The model under review builds one solid part; all positions refer to its coordinate system, in mm. A direction names the side the tool comes from. Give positions to 0.01 mm unless a question says otherwise; leave off trailing zeros. Order: outer loops, then holes, each group sorted by start corner. A loop starts at its lowest first (then second) coordinate and runs counter-clockwise, first axis right, second up. Notation, with made-up numbers: (54, 10) - (70, 10) arc R23 cw to (70, 32) - close; hole circle Ø4 at (-35.75, -19). An arc over 180 degrees is marked (long way). Write item = value, one per line. Start each with the question number.
1. Mouldability with a two-part tool opening along X and no side actions: class faces 4 (the flat face through (0, 0, 0)), 5 (the cylindrical face through (3.612, -3.312, 22.185)), 6 (the conical face through (-2.545, -1.372, 8.397)) as pulls with the +X half, pulls with the -X half, needs draft (parallel to the pull), parting line crosses it, or undercut.
2. We need section A-A, the plane z = 35. Give the boundary of the cut face in (x, y).
3. We need section D-D, the plane z = 5. Give the boundary of the cut face in (x, y).
4. We need section B-B, the plane z = 19. Give the boundary of the cut face in (x, y).
5. For P1, Ø2, axis at x = 2.5, y = 3.5, coming from the -Z side; P2, Ø1.4, axis at x = -2.6, y = -1.5, coming from the -Z side; P3, Ø1, axis at y = -4, z = 29, coming from the +X side; P4, Ø3.5, axis at x = 0, y = 0, coming from the +Z side, all flat-tipped, find the tip position at first contact; note any pin that passes through.
6. Machinability: for faces 1 (the cylindrical face through (-0.631, -2.003, 38.098)), 2 (the flat face through (-2.1, 1, 45)), 3 (the cylindrical face through (3.308, -1.131, 3.944)), which of the approach directions +Z, -Z, +X, -X, +Y, -Y give a long, thin tool a straight path to every point of the face, cutting with its end or side? Answer none if there is none.
7. Wall thickness on probe 1 along Y at (x, z) = (0, 4.25); probe 2 along X at (y, z) = (-1.75, 6); probe 3 along X at (y, z) = (3, 4): over which ranges is each line inside the solid? List them lowest first.
8. We need section C-C, the plane y = -3.25. Give the boundary of the cut face in (x, z).
from build123d import *

# Parameters (mm, degrees)
ESBO_O1_R                = 4.9
RESSALTO_EXTRUS_O1_DEPTH = 45
PADR_OCIRCULAR1_COUNT    = 3


with BuildPart() as part:
    # Esboço1 → Ressalto-extrusão1 (new body)
    with BuildSketch(Plane.XY):
        with Locations(Location((0, 0, 0), (0, 0, 180))):
            Circle(ESBO_O1_R)
    extrude(amount=RESSALTO_EXTRUS_O1_DEPTH)

    # Esboço2 → Furo roscado de M51 (revolve, cut)
    with BuildSketch(Plane(origin=(0, 0, 45), x_dir=(0, -1, 0), z_dir=(1, 0, 0))):
        Polygon((0, 0), (0, 15.2618073), (2.1, 14), (2.1, 0), align=None)
    revolve(axis=Axis((0, 0, 51.35), (0, 0, -1)), mode=Mode.SUBTRACT)

    # Esboço6 → Furo roscado de M21 (revolve, cut)
    with BuildSketch(Plane(origin=(0, 3, 0), x_dir=(0, 1, 0), z_dir=(1, 0, 0))):
        Polygon((0, 0), (0, 8.480688495), (0.8, 8), (0.8, 0), align=None)
    furo_roscado_de_m21 = revolve(axis=Axis((0, 3, -6.35), (0, 0, 1)), mode=Mode.SUBTRACT)

    # PadrãoCircular1: Furo roscado de M21 ×3 about axis
    padr_ocircular1_axis = Axis((0, 0, 0), (0, 0, 1))
    for i in range(1, PADR_OCIRCULAR1_COUNT):
        add(furo_roscado_de_m21.rotate(padr_ocircular1_axis, i * 360 / PADR_OCIRCULAR1_COUNT), mode=Mode.SUBTRACT)


solid = part.part
Model answer:
q1.face_4 = needs draft
q1.face_5 = parting line crosses it
q1.face_6 = undercut
q2.outline = circle Ø9.8 at (0, 0); hole circle Ø4.2 at (0, 0)
q3.outline = circle Ø9.8 at (0, 0); hole circle Ø1.6 at (-2.6, -1.5); hole circle Ø1.6 at (0, 3); hole circle Ø1.6 at (2.6, -1.5)
q4.outline = circle Ø9.8 at (0, 0)
q5.P1 = 0
q5.P2 = 8.06
q5.P3 = 3.43
q5.P4 = 30.79
q6.face_1 = +Z
q6.face_2 = +Z, +X, -X, +Y, -Y
q6.face_3 = -Z
q7.probe_1 = -4.9 to 2.2, 3.8 to 4.9
q7.probe_2 = -4.58 to -3.36, -1.84 to 1.84, 3.36 to 4.58
q7.probe_3 = -3.87 to -0.8, 0.8 to 3.87
q8.outline = (-3.67, 0) - (3.67, 0) - (3.67, 45) - (-3.67, 45) - close
